Source: CAD feature listing. Evaluate the final solid. Frame: model axes, mm. Give positions to 0.01 mm unless a question says otherwise; leave off trailing zeros. Loops run counter-clockwise (first coordinate to the right, second up) from the corner with the lowest first, then second, coordinate; pieces in that order, holes last. Notation, with made-up numbers: (76, 51) - (107, 51) arc R22 cw to (107, 86) - close; hole circle Ø1 at (-26.5, 0). An arc over 180 degrees is marked (long way). Put each result on its own line as item: value.
```python
from build123d import *

# Parameters (mm, degrees)
ESBO_O1_R                = 1.6
ESBO_O1_W                = 41
ESBO_O1_H                = 21
ESBO_O1_W_2              = 15
ESBO_O1_H_2              = 3
RESSALTO_EXTRUS_O1_DEPTH = 3
FILETE1_R                = 5
FILETE4_R                = 5


with BuildPart() as part:
    # Esboço1 → Ressalto-extrusão1 (new body)
    with BuildSketch(Plane.XY):
        Polygon((-30.5, 0.5), (-30.5, -19.5), (30.5, -19.5), (30.5, 0.5), (47.5, 0.5), (47.5, 10.5), (30.5, 10.5), (30.5, 19.5), (-19, 19.5), (-19, 36.5), (-30.5, 36.5), (-30.5, 10.5), (-42.5, 10.5), (-42.5, 0.5), align=None)
        with Locations((-24.75, 6.5)):
            Circle(ESBO_O1_R, mode=Mode.SUBTRACT)
        Rectangle(ESBO_O1_W, ESBO_O1_H, mode=Mode.SUBTRACT)
        with Locations((3, -14.5)):
            Rectangle(ESBO_O1_W_2, ESBO_O1_H_2, mode=Mode.SUBTRACT)
        with Locations((3, 14.5)):
            Rectangle(ESBO_O1_W_2, ESBO_O1_H_2, mode=Mode.SUBTRACT)
        with Locations((-37.5, 5.5)):
            Circle(ESBO_O1_R, mode=Mode.SUBTRACT)
        with Locations((42.5, 5.5)):
            Circle(ESBO_O1_R, mode=Mode.SUBTRACT)
        with Locations((-24.75, 31.5)):
            Circle(ESBO_O1_R, mode=Mode.SUBTRACT)
    extrude(amount=RESSALTO_EXTRUS_O1_DEPTH)

    # Filete1
    filete1_edges = [part.edges().sort_by_distance(p)[0] for p in [
        (-19, 36.5, 1.5),
        (-30.5, 36.5, 1.5),
        (30.5, -19.5, 1.5),
        (-30.5, -19.5, 1.5),
        (-42.5, 0.5, 1.5),
        (-19, 19.5, 1.5),
        (-30.5, 0.5, 1.5),
        (-30.5, 10.5, 1.5),
        (-42.5, 10.5, 1.5),
        (30.5, 0.5, 1.5),
        (47.5, 0.5, 1.5),
        (47.5, 10.5, 1.5),
        (30.5, 10.5, 1.5),
    ]]
    fillet(filete1_edges, radius=FILETE1_R - 0.0001)  # a hair under: the kernel refuses the full size

    # Filete4
    filete4_edges = [part.edges().sort_by_distance(p)[0] for p in [
        (30.5, 19.5, 1.5),
    ]]
    fillet(filete4_edges, radius=FILETE4_R)


solid = part.part
```
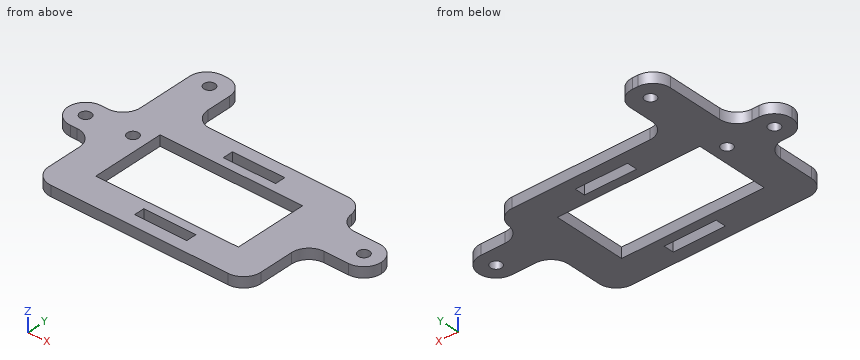
1) Material intervals for line 1 along Y through (x, z) = (-24.75, 1); line 2 along Y through (x, z) = (42.5, 1.1); line 3 along Y through (x, z) = (-7, 1.15), sorted ascending. Write a range as [from, to].
Check result:
line 1: [-19.5, 4.9], [8.1, 29.9], [33.1, 36.5]
line 2: [0.5, 3.9], [7.1, 10.5]
line 3: [-19.5, -10.5], [10.5, 19.5]
2) Section query D-D, the plane z = 0.8. State how many separate pieces and enclosed holes the cut face has, plus the area to 3 significant figures.
Check result:
separate pieces: 1
enclosed holes: 7
area: 1,860 mm²
3) Pin query (flat end, axial travel): P1, Ø1.5, axis at y = 20.5, z = 1.5, coming from the -X side; P2, Ø1.5, axis at y = 15, z = 1, coming from the +X side; P3, Ø0.9, axis at x = 39.5, z = 1.5, coming from the -Y side. Return the tip coordinate at first contact, or that it passes through.
Check result:
P1: x = -30.5
P2: x = 30.66
P3: y = 0.5
4) Section query B-B, the plane x = -10.5. Output: boundary loops of the cut face in (y, z).
Check result:
outline: (-19.5, 0) - (-10.5, 0) - (-10.5, 3) - (-19.5, 3) - close; (10.5, 0) - (19.5, 0) - (19.5, 3) - (10.5, 3) - close
5) Section query A-A, the plane x = 7.5. Output: boundary loops of the cut face in (y, z).
Check result:
outline: (-19.5, 0) - (-16, 0) - (-16, 3) - (-19.5, 3) - close; (-13, 0) - (-10.5, 0) - (-10.5, 3) - (-13, 3) - close; (10.5, 0) - (13, 0) - (13, 3) - (10.5, 3) - close; (16, 0) - (19.5, 0) - (19.5, 3) - (16, 3) - close
6) Section query C-C, the plane y = -2.5. Output: boundary loops of the cut face in (x, z).
Check result:
outline: (-30.92, 0) - (-20.5, 0) - (-20.5, 3) - (-30.92, 3) - close; (20.5, 0) - (30.92, 0) - (30.92, 3) - (20.5, 3) - close
